The drawing under review shows one solid part. Ordinate dimensions are in mm from its lowest x, y, z. Round coordinates to 2 decimals unless told otherwise and drop trailing zeros. Write each loop counter-clockwise with the first axis right and the second up, starting at its lowest first coordinate (ties: lowest second). Pieces come first, ordered by that corner, then holes. Notation, with made-up numbers: (87, 42.25) -> (113, 42.25) arc R20 cw to (113, 72.25) -> close; hole circle Ø5 at (57, 12). An arc over 180 degrees is marked (long way). Answer in a Markdown table with one row per item.
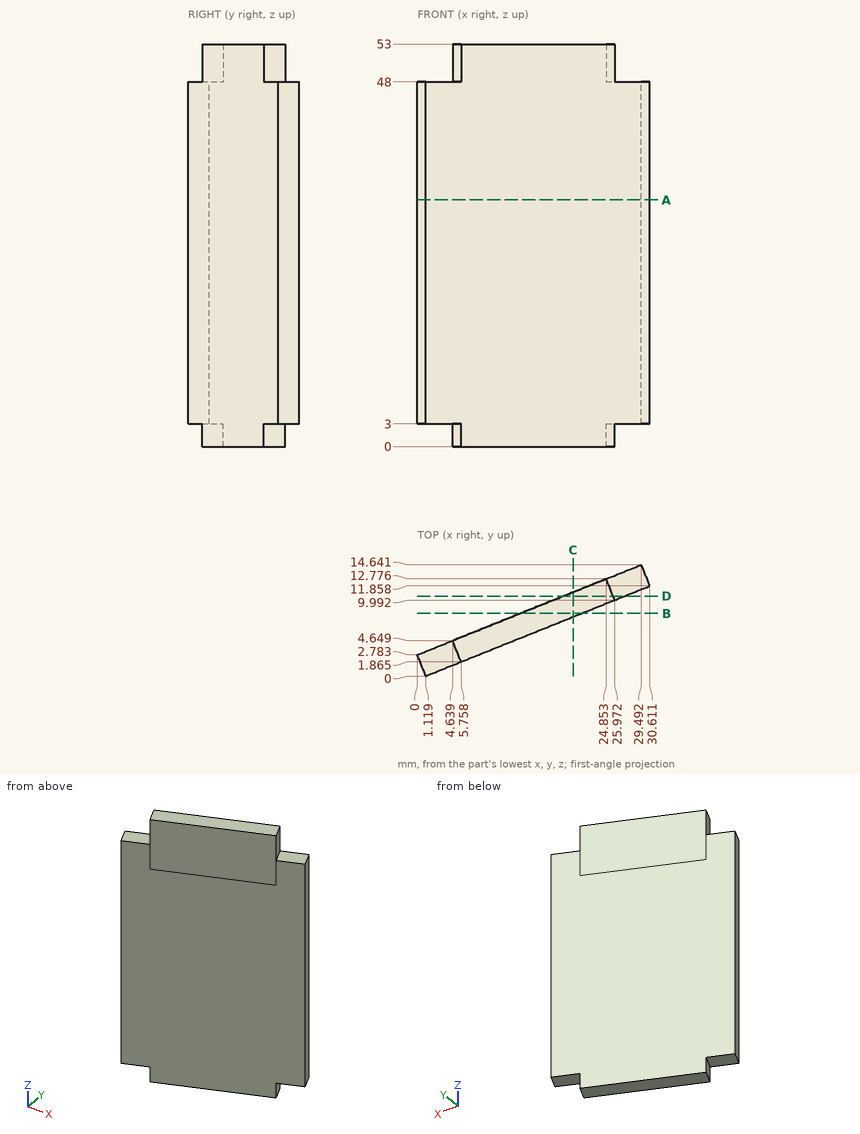
1) Consider section C-C on x = 20.5. State the section outline as (y, z) points (1 decimal).
Solved:
| item | result |
|---|---|
| outline | (7.8, 0) -> (11, 0) -> (11, 53) -> (7.8, 53) -> close |
2) Consider section B-B on y = 8.25. State the section outline as (x, z) points.
Solved:
| item | result |
|---|---|
| outline | (13.6, 0) -> (21.64, 0) -> (21.64, 53) -> (13.6, 53) -> close |
3) For line 1 (Z direction, x = 5.5, y = 2.25); line 2 (X direction, y = 3.5, z = 50.5) (1 decimal); line 3 (X direction, y = 11, z = 27) (1 decimal), list the stretches that pass through material, from the lowest coordinate up. Write a range as [from, to].
Solved:
| item | result |
|---|---|
| line 1 | [3, 48] |
| line 2 | [5.1, 9.8] |
| line 3 | [20.4, 28.5] |
4) Consider section A-A on z = 32.5. State the section outline as (x, y) points.
Solved:
| item | result |
|---|---|
| outline | (0, 2.78) -> (1.12, 0) -> (30.61, 11.86) -> (29.49, 14.64) -> close |
5) Clearance check with flat-ended pins moving along their axes: pin 1 Ø2.5 at (x, y) = (2.5, 2.5) entering from -Z; pin 2 Ø10 at (x, z) = (22.5, 10) entering from -Y; pin 3 Ø12 at (x, z) = (26.5, 12.5) entering from -Y. State where each tip first meets the part, or that it passes through.
Solved:
| item | result |
|---|---|
| pin 1 | z = 3 |
| pin 2 | y = 6.59 |
| pin 3 | y = 7.79 |
6) Consider section D-D on y = 10.5. State the section outline as (x, z) points (1 decimal).
Solved:
| item | result |
|---|---|
| outline | (19.2, 0) -> (25.8, 0) -> (25.8, 3) -> (27.2, 3) -> (27.2, 48) -> (25.8, 48) -> (25.8, 53) -> (19.2, 53) -> close |
